Job drawing, mm, ordinate dimensions from the low corner. One solid piece. A direction names the side the tool comes from. Coordinates: 2 decimals unless noted, no trailing zeros. Write each loop counter-clockwise with the first axis right and the second up, starting at its lowest first coordinate (ties: lowest second). Pieces come first, ordered by that corner, then holes. Notation, with made-up numbers: (-20, 54) - (33, 54) arc R25 ccw to (33, 68) - close; hole circle Ø10 at (34.25, 22.25). An arc over 180 degrees is marked (long way). Use a Markdown table: item, result.
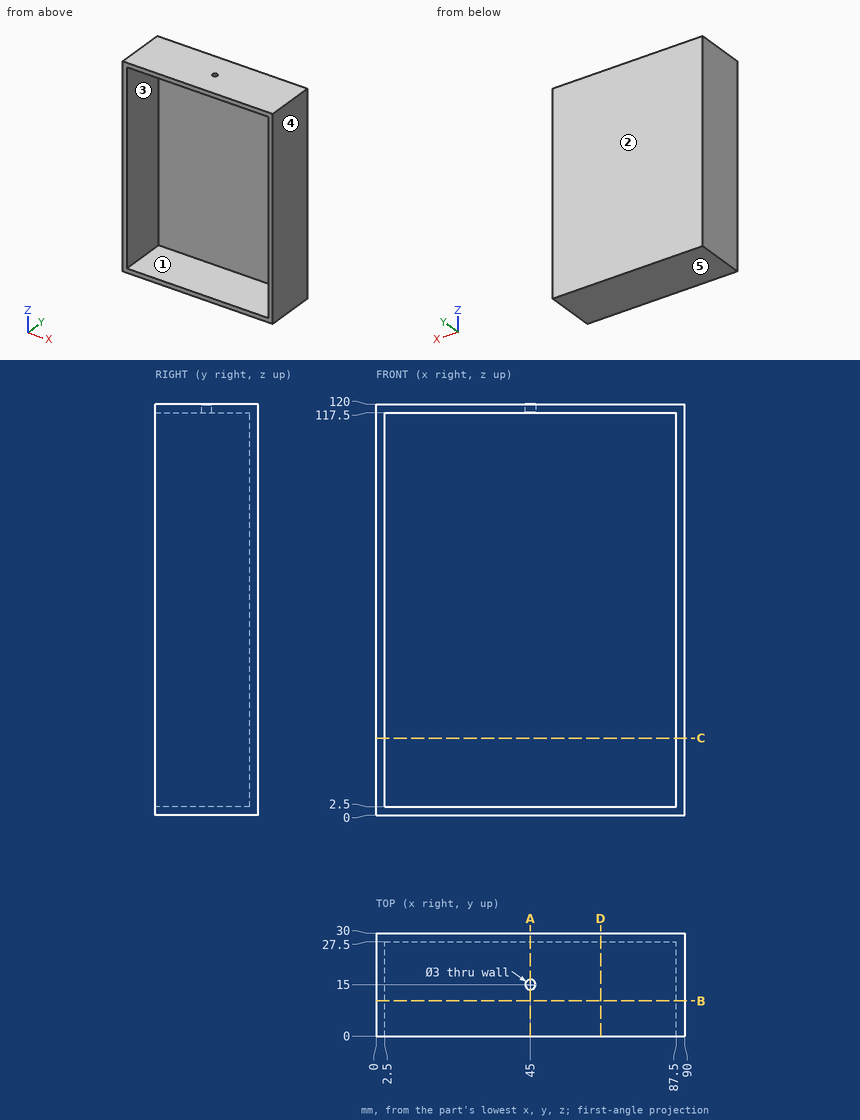
Item 1: Which spindle directions (+Z, -Z, +X, -X, +Y, -Y) get a long thin tool onto all of the face, cutting with end or side? Do the marked faces 1 and 2. Say none if no direction does.
From the geometry:
| item | result |
|---|---|
| face 1 | -Y |
| face 2 | +Z, -Z, +X, -X, +Y |
Item 2: Band-saw the part on A-A, the plane x = 45. Give the cut face in (y, z), then the cut area to 3 significant figures.
From the geometry:
| item | result |
|---|---|
| outline | (0, 0) - (30, 0) - (30, 120) - (16.5, 120) - (16.5, 117.5) - (27.5, 117.5) - (27.5, 2.5) - (0, 2.5) - close; (0, 117.5) - (13.5, 117.5) - (13.5, 120) - (0, 120) - close |
| area | 430 mm^2 |
Item 3: Drill centre lines: probe 1 along Z at (x, y) = (85.5, 10); probe 2 along Y at (x, z) = (45, 118); probe 3 along X at (y, z) = (13, 91). Where is each one in solid material? Low to high.
From the geometry:
| item | result |
|---|---|
| probe 1 | 0 to 2.5, 117.5 to 120 |
| probe 2 | 0 to 13.5, 16.5 to 30 |
| probe 3 | 0 to 2.5, 87.5 to 90 |
Item 4: Band-saw the part on D-D, the plane x = 65.5. Give the cut face in (y, z).
From the geometry:
| item | result |
|---|---|
| outline | (0, 0) - (30, 0) - (30, 120) - (0, 120) - (0, 117.5) - (27.5, 117.5) - (27.5, 2.5) - (0, 2.5) - close |
Item 5: Band-saw the part on C-C, the plane z = 22.5. Give the cut face in (x, y), then the cut area to 4 significant figures.
From the geometry:
| item | result |
|---|---|
| outline | (0, 0) - (2.5, 0) - (2.5, 27.5) - (87.5, 27.5) - (87.5, 0) - (90, 0) - (90, 30) - (0, 30) - close |
| area | 362.5 mm^2 |
Item 6: Drop a flat-ended pin along its axis: P1, Ø5, axis at x = 62, z = 106, coming from the -Y side. Give the stop position or say it passes through.
From the geometry:
| item | result |
|---|---|
| P1 | y = 27.5 |
Item 7: Band-saw the part on B-B, the plane y = 10.25. Give the cut face in (x, z).
From the geometry:
| item | result |
|---|---|
| outline | (0, 0) - (90, 0) - (90, 120) - (0, 120) - close; hole (2.5, 2.5) - (87.5, 2.5) - (87.5, 117.5) - (2.5, 117.5) - close |
Item 8: Two-plate mould, pull along Z, no slides. Class the marked faces 3, 4 and 5: pulls with the +Z half, pulls with the -Z half, needs draft (parallel to the pull), parting line crosses it, or undercut.
From the geometry:
| item | result |
|---|---|
| face 3 | undercut |
| face 4 | needs draft |
| face 5 | pulls with the -Z half |
